Input: part model. Units: mm. Frame: model coordinates. Face numbers are marked on the shaded views. Coordinates: 2 decimals unless noted, no trailing zeros. Order: outer loops, then holes, each group sorted by start corner. A loop starts at its lowest first (then second) coordinate and runs counter-clockwise, first axis right, second up.
from build123d import *

# Parameters (mm, degrees)
F0_W     = 70
F0_H     = 30
F1_DEPTH = 8
F2_D     = 3.2
F3_D     = 12.5
F5_D     = 3.5
F5_DEPTH = 50
F5_TIP   = 1.0515060833
F6_D     = 4.4
F6_DEPTH = 15
F6_TIP   = 1.3218933619
F7_R     = 1.7108756352
F8_DEPTH = 3.456151576


with BuildPart() as f1:
    # F0 (on Top) → F1 (new body)
    with BuildSketch(Plane.XY):
        Rectangle(F0_W, F0_H)
    extrude(amount=-F1_DEPTH)

    # F2 (through all)
    with Locations(Plane.XY):
        with Locations((-28, 8), (-12, 8), (-28, -8), (-12, -8), (0, 8), (0, -8), (12, 8), (12, -8), (28, 8), (28, -8)):
            Hole(F2_D / 2)

    # F3 (through all)
    with Locations(Plane.XY):
        with Locations((-20, 0)):
            Hole(F3_D / 2)

    # F5
    with Locations(Plane.YZ.offset(35)):
        with Locations((0, -4)):
            Hole(F5_D / 2, depth=F5_DEPTH)
            with Locations((0, 0, -(F5_DEPTH + F5_TIP / 2))):  # 118° drill point
                Cone(0, F5_D / 2, F5_TIP, mode=Mode.SUBTRACT)

    # F6
    with Locations(Plane.YZ.offset(35)):
        with Locations((0, -4)):
            Hole(F6_D / 2, depth=F6_DEPTH)
            with Locations((0, 0, -(F6_DEPTH + F6_TIP / 2))):  # 118° drill point
                Cone(0, F6_D / 2, F6_TIP, mode=Mode.SUBTRACT)

    # F7 (on face) → F8 (cut, through all)
    with BuildSketch(Plane(origin=(0, 0, -8), x_dir=(1, 0, 0), z_dir=(0, 0, -1))):
        with Locations((20.1314277947, 0)):
            Circle(F7_R)
    extrude(amount=-F8_DEPTH, mode=Mode.SUBTRACT)


solid = f1.part
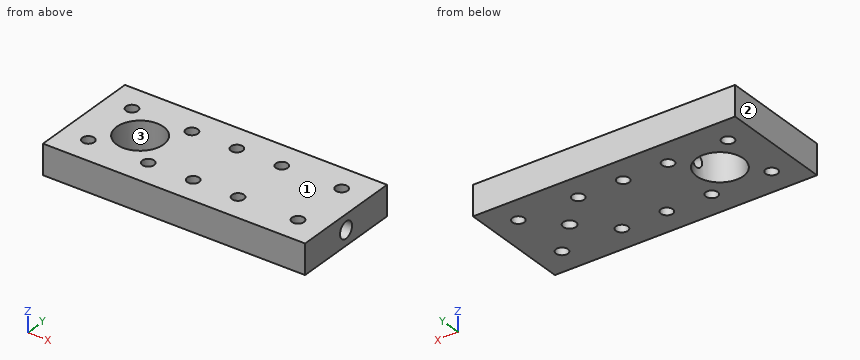
Item 1: Cut plane A-A on x = -28. Return loops of the section in (y, z), then the cut area to 3 significant figures.
Response values:
outline: (-15, -8) - (-9.6, -8) - (-9.6, 0) - (-15, 0) - close; (-6.4, -8) - (6.4, -8) - (6.4, 0) - (-6.4, 0) - close; (9.6, -8) - (15, -8) - (15, 0) - (9.6, 0) - close
area: 189 mm2
Item 2: Ray query, probe 1 along Y at (x, z) = (12, -4); probe 2 along X at (y, z) = (-7.25, -6); probe 3 along Y at (x, z) = (24, -4). Return the intervals inside material, ascending.
Response values:
probe 1: y = -15 to -9.6, -6.4 to -1.75, 1.75 to 6.4, 9.6 to 15
probe 2: x = -35 to -29.41, -26.59 to -13.41, -10.59 to -1.41, 1.41 to 10.59, 13.41 to 26.59, 29.41 to 35
probe 3: y = -15 to -2.2, 2.2 to 15
Item 3: Draft query along X for the marked faces 1, 2 and 3. Return one class per face: pulls with the +X half, pulls with the -X half, needs draft (parallel to the pull), parting line crosses it, or undercut.
Response values:
face 1: needs draft
face 2: pulls with the -X half
face 3: undercut
Item 4: Cut plane C-C on x = -12. Return loops of the section in (y, z).
Response values:
outline: (-15, -8) - (-9.6, -8) - (-9.6, 0) - (-15, 0) - close; (-6.4, -8) - (6.4, -8) - (6.4, 0) - (-6.4, 0) - close; (9.6, -8) - (15, -8) - (15, 0) - (9.6, 0) - close; hole circle Ø3.5 at (0, -4)
Item 5: Pin query (flat end, axial travel): pin 1 Ø3 at (x, y) = (-12, 8) entering from -Z. Return the tip coordinate at first contact, or that it passes through.
Response values:
pin 1: passes through
Item 6: Cut plane D-D on z = -1. Count the separate pieces of the cut face and the enclosed holes in it, then the cut area to 3 significant figures.
Response values:
separate pieces: 1
enclosed holes: 11
area: 1,900 mm2
Item 7: Cut plane B-B on y = 8. Return loops of the section in (x, z), then the cut area to 3 significant figures.
Response values:
outline: (-35, -8) - (-29.6, -8) - (-29.6, 0) - (-35, 0) - close; (-26.4, -8) - (-13.6, -8) - (-13.6, 0) - (-26.4, 0) - close; (-10.4, -8) - (-1.6, -8) - (-1.6, 0) - (-10.4, 0) - close; (1.6, -8) - (10.4, -8) - (10.4, 0) - (1.6, 0) - close; (13.6, -8) - (26.4, -8) - (26.4, 0) - (13.6, 0) - close; (29.6, -8) - (35, -8) - (35, 0) - (29.6, 0) - close
area: 432 mm2
